Source: CAD feature listing. Evaluate the final solid. Frame: model axes, mm. Give positions to 0.01 mm unless a question says otherwise; leave off trailing zeros. Order: outer loops, then holes, each group sorted by start corner. A loop starts at its lowest first (then second) coordinate and runs counter-clockwise, first axis right, second up.
```python
from build123d import *

# Parameters (mm, degrees)
BOSS_EXTRU_1_DEPTH = 10
BOSS_EXTRU_2_DEPTH = 10


with BuildPart() as part:
    # Esquisse1 → Boss.-Extru.1 (new body)
    with BuildSketch(Plane(origin=(0, 0, 0), x_dir=(1, 0, 0), z_dir=(0, 1, 0))):
        with BuildLine():
            Line((10, 45.412002819), (10, 35.103418637))
            ThreePointArc((10, 35.103418637), (-21.991475621, 29.131168875), (-36.5, 0))
            Line((-36.5, 0), (-46.5, 0))
            ThreePointArc((-46.5, 0), (-29.131168875, 36.243965015), (10, 45.412002819))
        make_face()
    extrude(amount=BOSS_EXTRU_1_DEPTH)

    # Esquisse4 → Boss.-Extru.2 (add)
    with BuildSketch(Plane(origin=(0, 10, 0), x_dir=(1, 0, 0), z_dir=(0, 1, 0))):
        with BuildLine():
            Line((-36.5, 0), (-46.5, 0))
            Line((-46.5, 0), (-46.5, -30.702684518))
            Line((-46.5, -30.702684518), (-58.034822919, -59.225728707))
            Line((-58.034822919, -59.225728707), (-91.599603917, -39.502076956))
            ThreePointArc((-91.599603917, -39.502076956), (-98.443575905, -41.279729178), (-96.665923684, -48.123701166))
            Line((-96.665923684, -48.123701166), (-53.109165443, -73.7189324))
            Line((-53.109165443, -73.7189324), (-36.5, -32.648170999))
            Line((-36.5, -32.648170999), (-36.5, 0))
        make_face()
    extrude(amount=-BOSS_EXTRU_2_DEPTH)


solid = part.part
```
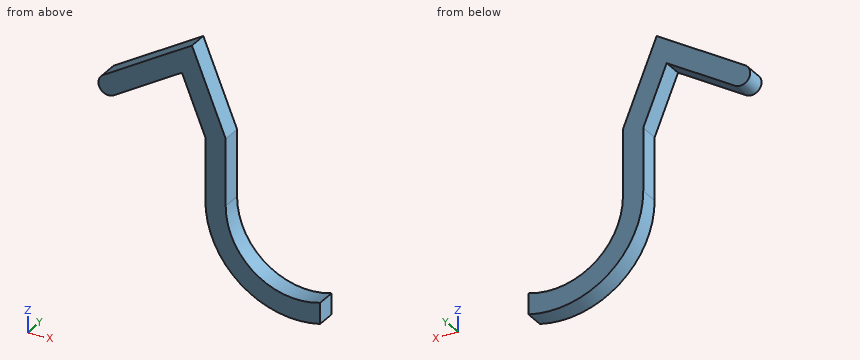
1) Section query B-B, the plane z = 50.5. Return the cut outline in (x, y), and give its area (3 significant figures).
Report:
outline: (-92.62, 0) - (-72.88, 0) - (-72.88, 10) - (-92.62, 10) - close; (-54.51, 0) - (-43.72, 0) - (-43.72, 10) - (-54.51, 10) - close
area: 305 mm2
2) Section query C-C, the plane z = 7. Return the cut outline in (x, y), and give its area (3 significant figures).
Report:
outline: (-46.5, 0) - (-36.5, 0) - (-36.5, 10) - (-46.5, 10) - close
area: 100 mm2
3) Section query A-A, the plane y = 8. Return the cut outline in (x, z).
Report:
outline: (-96.67, 48.12) arc R5 ccw to (-91.6, 39.5) - (-58.03, 59.23) - (-46.5, 30.7) - (-46.5, 0) arc R46.5 ccw to (10, -45.41) - (10, -35.1) arc R36.5 cw to (-36.5, 0) - (-36.5, 32.65) - (-53.11, 73.72) - close
4) Pin query (flat end, axial travel): pin 1 (3 mm diameter, centred on x = -4.5, y = 5.5, fed in from +Z); pin 2 (3 mm diameter, centred on y = 3, z = 16.5, fed in from +X); pin 3 (3 mm diameter, centred on y = 5.5, z = 41, fed in from +X). Return the tip coordinate at first contact, or that it passes through.
Report:
pin 1: stops at z = -36
pin 2: stops at x = -36.5
pin 3: stops at x = -39.27
5) Material intervals for L1, parallel to Z at x = 1, y = 3; L2, parallel to X at y = 3.75, z = 6; L3, parallel to X at y = 5.75, z = 57, sorted ascending.
Report:
L1: z = -46.49 to -36.49
L2: x = -46.5 to -36.5
L3: x = -81.56 to -61.82, -57.13 to -46.35
6) Section query D-D, the plane x = -55.5. Return the cut outline in (y, z), and give its area (3 significant figures).
Report:
outline: (0, 52.96) - (10, 52.96) - (10, 72.31) - (0, 72.31) - close
area: 194 mm2
